CAD build for the part. Positions are in the model's coordinates, mm. Face numbers are marked on the shaded views. A direction names the side the tool comes from. Round coordinates to 2 decimals unless told otherwise and drop trailing zeros. Order: outer loops, then holes, each group sorted by start corner. A loop starts at its lowest first (then second) coordinate and runs counter-clockwise, first axis right, second up. Notation, with made-up numbers: M 81.5,-39 L 103.5,-39 A35 cw 103.5,-5 Z; hole C 85.5,12.5 d9. An arc over 180 degrees is marked long. Answer as a JSON object with one key per item and string values. Group by question number.
```python
from build123d import *

# Parameters (mm, degrees)
ESBO_O1_R                     = 1.6
RESSALTO_EXTRUS_O1_DEPTH      = 3
RESSALTO_EXTRUS_O1_2_DEPTH    = 3
RESSALTO_EXTRUS_O2_DEPTH      = 8
RESSALTO_EXTRUS_O2_DEPTH_BACK = 3
CORTE_EXTRUS_O1_DEPTH         = 26.357444666
CORTE_EXTRUS_O1_DEPTH_BACK    = 26.357444666
ESBO_O3_R                     = 1.65


with BuildPart() as part:
    # Esbo_o1 → Ressalto-extrus_o1 (new body)
    with BuildSketch(Plane.XY):
        with BuildLine():
            ThreePointArc((-4, -0.9), (-0.051399019, -4.099677809), (3.97617907, -1))
            Line((3.97617907, -1), (8, -1))
            Line((8, -1), (8, -15))
            Line((8, -15), (-4, -15))
            Line((-4, -15), (-4, -0.9))
        make_face()
        with Locations((2, -11)):
            Circle(ESBO_O1_R, mode=Mode.SUBTRACT)
    extrude(amount=RESSALTO_EXTRUS_O1_DEPTH)



with BuildPart() as body_2:
    # Esbo_o1 → Ressalto-extrus_o1 2 (new body)
    with BuildSketch(Plane.XY):
        with BuildLine():
            ThreePointArc((3.97617907, 1), (-0.051399019, 4.099677809), (-4, 0.9))
            Line((-4, 0.9), (-4, 15))
            Line((-4, 15), (8, 15))
            Line((8, 15), (8, 1))
            Line((8, 1), (3.97617907, 1))
        make_face()
        with Locations((2, 11)):
            Circle(ESBO_O1_R, mode=Mode.SUBTRACT)
    extrude(amount=RESSALTO_EXTRUS_O1_2_DEPTH)


with BuildPart() as part_1:
    add(part.part)

    add(body_2.part)  # Ressalto-extrus_o2 merges body 2
    # Esbo_o2 → Ressalto-extrus_o2 (add, two sides: drawn at the far end of the back side and taken through both)
    with BuildSketch(Plane.XY.offset(3).offset(-RESSALTO_EXTRUS_O2_DEPTH_BACK)):
        with BuildLine():
            Line((9, 6), (9, 1))
            Line((9, 1), (3.97617907, 1))
            ThreePointArc((3.97617907, 1), (-4.1, 0), (3.97617907, -1))
            Line((3.97617907, -1), (9, -1))
            Line((9, -1), (9, -6))
            Line((9, -6), (0, -6))
            ThreePointArc((0, -6), (-6, 0), (0, 6))
            Line((0, 6), (9, 6))
        make_face()
    extrude(amount=RESSALTO_EXTRUS_O2_DEPTH + RESSALTO_EXTRUS_O2_DEPTH_BACK)

    # Esbo_o3 → Corte-extrus_o1 (cut, two sides: drawn at the far end of the back side and taken through both)
    with BuildSketch(Plane.XZ.offset(-6).offset(-CORTE_EXTRUS_O1_DEPTH_BACK)):
        with Locations(Location((6.6, 7, 0), (0, 0, 270))):
            Circle(ESBO_O3_R)
    extrude(amount=CORTE_EXTRUS_O1_DEPTH + CORTE_EXTRUS_O1_DEPTH_BACK, mode=Mode.SUBTRACT)


solid = part_1.part
```
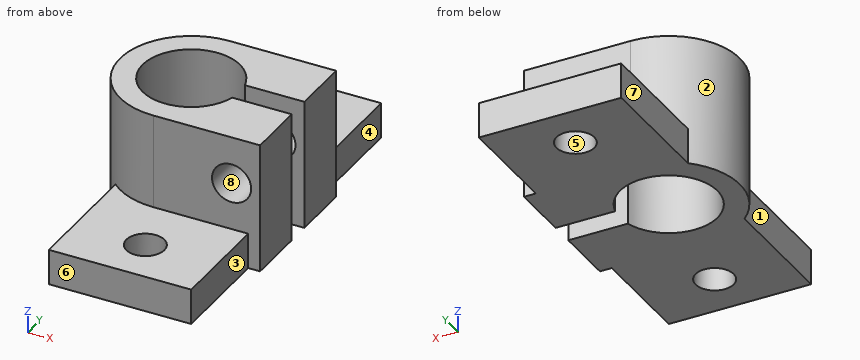
Item 1: Cut at A-A, the plane y = 11. Give the cut face in (x, z).
Item 2: Two-plate mould, pull along X, no slides. Class the marked faces 5, 6, 7 and 8: +X half, -X half, draft (parallel to the pull), parting line (faces both ways), or undercut.
Item 3: Cut at C-C, the plane x = 3.25. Give the cut face in (y, z).
Item 4: Drill centre lines: line 1 (Y direction, x = 2, z = 1.6); line 2 (Y direction, x = 8.25, z = 7.5); line 3 (X direction, y = -2.9, z = 7). Where is each one in solid material? Low to high. Write a range as [from, to].
Item 5: Cut at D-D, the plane z = 1.5. Give the cut face in (x, y), and give its area (3 significant figures).
Item 6: Flat gauge pins, fed straight in: pin 1 Ø2.5 at (x, z) = (5.5, 6.5) entering from +Y; pin 2 Ø8.5 at (x, y) = (2, -9) entering from +Z; pin 3 Ø0.9 at (y, z) = (-12, 1.5) entering from +X; pin 4 Ø1.5 at (y, z) = (12.5, 2) entering from -X. Where does each tip first touch, or does it go through?
Item 7: Cut at B-B, the plane z = 7. Give the cut face in (x, y), and give its area (3 significant figures).
Item 8: 3-axis set-ups, long thin cutter, end or side, ignore diameter. For the marked faces 1, 2, 3 and 4: which of +Z, -Z, +X, -X, +Y, -Y reach the whole face in a straight line?
Response values:
{
 "1": {"outline": "M -4,0 L 0.4,0 L 0.4,3 L -4,3 Z; M 3.6,0 L 8,0 L 8,3 L 3.6,3 Z"},
 "2": {"face 5": "undercut", "face 6": "draft", "face 7": "-X half", "face 8": "undercut"},
 "3": {"outline": "M -15,0 L -12,0 L -12,3 L -15,3 Z; M -10,0 L -2.5,0 L -2.5,11 L -6,11 L -6,3 L -10,3 Z; M 2.5,0 L 10,0 L 10,3 L 6,3 L 6,11 L 2.5,11 Z; M 12,0 L 15,0 L 15,3 L 12,3 Z"},
 "4": {"line 1": "[-15, -12.6], [-9.4, -3.58], [3.58, 9.4], [12.6, 15]", "line 2": "[-6, -1], [1, 6]", "line 3": "[-5.25, -2.9], [2.9, 4.95], [8.25, 9]"},
 "5": {"outline": "M -4,-15 L 8,-15 L 8,-6 L 9,-6 L 9,-1 L 3.98,-1 A4.1 cw long 3.98,1 L 9,1 L 9,6 L 8,6 L 8,15 L -4,15 L -4,4.47 A6 ccw -4,-4.47 Z; hole C 2,-11 d3.2; hole C 2,11 d3.2", "area": "306 mm^2"},
 "6": {"pin 1": "y = 6", "pin 2": "z = 11", "pin 3": "x = 8", "pin 4": "x = -4"},
 "7": {"outline": "M 0,-6 L 4.95,-6 L 4.95,-1 L 3.98,-1 A4.1 cw long 3.98,1 L 4.95,1 L 4.95,6 L 0,6 A6 ccw Z; M 8.25,-6 L 9,-6 L 9,-1 L 8.25,-1 Z; M 8.25,1 L 9,1 L 9,6 L 8.25,6 Z", "area": "68.9 mm^2"},
 "8": {"face 1": "+Z, -Z, -X, -Y", "face 2": "+Z, -X", "face 3": "+Z, -Z, +X, -Y", "face 4": "+Z, -Z, +X, +Y"}
}
